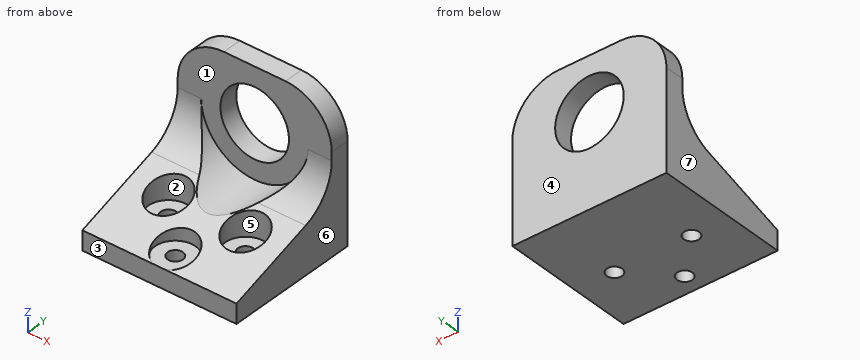
from build123d import *

# Parameters (mm, degrees)
SKETCH1_W           = 50.8
SKETCH1_H           = 44.45
BOSS_EXTRUDE1_DEPTH = 6.35
BOSS_EXTRUDE2_DEPTH = 50.8
SKETCH3_R           = 11.303
CUT_EXTRUDE1_DEPTH  = 50.8
SKETCH4_R           = 2.54
CUT_EXTRUDE2_DEPTH  = 50.8
SKETCH5_R           = 6.6675
CUT_EXTRUDE3_DEPTH  = 41.656
SKETCH6_R           = 17.653
CUT_EXTRUDE4_DEPTH  = 50.8
FILLET1_R           = 15.24


with BuildPart() as part:
    # Sketch1 → Boss-Extrude1 (new body)
    with BuildSketch(Plane.XY):
        with Locations((25.4, 22.225)):
            Rectangle(SKETCH1_W, SKETCH1_H)
    extrude(amount=BOSS_EXTRUDE1_DEPTH)

    # Sketch2 → Boss-Extrude2 (add)
    with BuildSketch(Plane(origin=(50.8, 0, 0), x_dir=(0, 0, -1), z_dir=(1, 0, 0))):
        Polygon((-6.35, 0), (-6.35, 44.45), (-48.006, 44.45), (-48.006, 38.1), (-19.05, 38.1), align=None)
    extrude(amount=-BOSS_EXTRUDE2_DEPTH)

    # Sketch3 → Cut-Extrude1 (cut)
    with BuildSketch(Plane(origin=(0, 44.45, 0), x_dir=(1, 0, 0), z_dir=(0, 1, 0))):
        with Locations(Location((25.4, -30.353, 0), (0, 0, 270))):
            Circle(SKETCH3_R)
    extrude(amount=-CUT_EXTRUDE1_DEPTH, mode=Mode.SUBTRACT)

    # Sketch4 → Cut-Extrude2 (cut)
    with BuildSketch(Plane(origin=(0, 0, 0), x_dir=(-1, 0, 0), z_dir=(0, 0, -1))):
        with Locations((-25.4, 6.35)):
            Circle(SKETCH4_R)
        with Locations((-38.1, 19.05)):
            Circle(SKETCH4_R)
        with Locations((-12.7, 19.05)):
            Circle(SKETCH4_R)
    extrude(amount=-CUT_EXTRUDE2_DEPTH, mode=Mode.SUBTRACT)

    # Sketch5 → Cut-Extrude3 (cut)
    with BuildSketch(Plane.XY.offset(48.006)):
        with Locations((12.7, 19.05)):
            Circle(SKETCH5_R)
        with Locations((38.1, 19.05)):
            Circle(SKETCH5_R)
        with Locations((25.4, 6.35)):
            Circle(SKETCH5_R)
    extrude(amount=-CUT_EXTRUDE3_DEPTH, mode=Mode.SUBTRACT)

    # Sketch6 → Cut-Extrude4 (cut)
    with BuildSketch(Plane.XZ.offset(-38.1)):
        with Locations((25.4, 30.353)):
            Circle(SKETCH6_R)
    extrude(amount=CUT_EXTRUDE4_DEPTH, mode=Mode.SUBTRACT)

    # Fillet1
    fillet1_edges = [part.edges().sort_by_distance(p)[0] for p in [
        (5.92005531, 38.1, 19.05),
        (44.87994469, 38.1, 19.05),
        (50.8, 41.275, 48.006),
        (0, 41.275, 48.006),
    ]]
    fillet(fillet1_edges, radius=FILLET1_R)


solid = part.part
Geometry check sheet. Reference: the model listing, model coordinates, mm. Face numbers are marked on the shaded views. A direction names the side the tool comes from. Give positions to 0.01 mm unless a question says otherwise; leave off trailing zeros. Loops run counter-clockwise (first coordinate to the right, second up) from the corner with the lowest first, then second, coordinate; pieces in that order, holes last. Notation, with made-up numbers: (-22.75, 41.5) -> (28.25, 41.5) arc R23 cw to (28.25, 72.5) -> close; hole circle Ø1 at (74.5, 14.25). An arc over 180 degrees is marked (long way). Answer in a Markdown table with one row per item. Add a question column.
1) Set-up check for the marked faces 1, 2 and 3: record each of +Z, -Z, +X, -X, +Y, -Y from which the full face is reachable in a straight line by a thin tool's end or side.
2) Material ranges on probe 1 along X at (y, z) = (19.05, 11.75); probe 2 along X at (y, z) = (19, 4); probe 3 along X at (y, z) = (6, 7), recorded low to high. Write a range as from..to.
3) Cross-section at C-C on z = 23. Record the boundary of the cut face in (x, y), and give its area (3 significant figures).
4) Gauge pin test, flat ends, axial feed: P1, Ø12, axis at y = 9, z = 18.5, coming from the +X side; P2, Ø3, axis at x = 39, y = 12, coming from the -Z side; P3, Ø4, axis at x = 17.5, y = 22, coming from the +Z side; P4, Ø1, axis at x = 45.5, y = 28, coming from the +Z side. Record the tip position at first contact, or that the pin passes through.
5) Cross-section at A-A on x = 25.4. Record the boundary of the cut face in (y, z), and give its area (3 significant figures).
6) Cross-section at B-B on y = 6.35. Record the boundary of the cut face in (x, z), and give its area (3 significant figures).
7) Draft check along X on the marked faces 4, 5, 6 and 7. Enter one of: pulls with the +X half, pulls with the -X half, needs draft (parallel to the pull), parting line crosses it, or undercut.
8) Cross-section at D-D on x = 38.1. Record the boundary of the cut face in (y, z).
Outcome:
| question | item | result |
|---|---|---|
| 1 | face 1 | +Z, -Y |
| 1 | face 2 | +Z |
| 1 | face 3 | +Z, -Z, +X, -X, -Y |
| 2 | probe 1 | x = 0..6.03, 19.37..31.43, 44.77..50.8 |
| 2 | probe 2 | x = 0..10.16, 15.24..35.56, 40.64..50.8 |
| 2 | probe 3 | x = 0..18.74, 32.06..50.8 |
| 3 | outline | (0, 36.38) -> (9.35, 36.38) -> (9.35, 38.1) -> (16.82, 38.1) -> (16.82, 44.45) -> (0, 44.45) -> close; (33.98, 38.1) -> (41.45, 38.1) -> (41.45, 36.38) -> (50.8, 36.38) -> (50.8, 44.45) -> (33.98, 44.45) -> close |
| 3 | area | 246 mm^2 |
| 4 | P1 | passes through |
| 4 | P2 | stops at z = 0 |
| 4 | P3 | stops at z = 14.35 |
| 4 | P4 | stops at z = 15.88 |
| 5 | outline | (0, 0) -> (3.81, 0) -> (3.81, 6.35) -> (0, 6.35) -> close; (8.89, 0) -> (44.45, 0) -> (44.45, 19.05) -> (38.1, 19.05) -> (38.1, 12.7) -> (19.05, 12.7) -> (13.02, 10.69) -> (13.02, 6.35) -> (8.89, 6.35) -> close; (38.1, 41.66) -> (44.45, 41.66) -> (44.45, 48.01) -> (38.1, 48.01) -> close |
| 5 | area | 524 mm^2 |
| 6 | outline | (0, 0) -> (22.86, 0) -> (22.86, 6.35) -> (18.73, 6.35) -> (18.73, 8.47) -> (0, 8.47) -> close; (27.94, 0) -> (50.8, 0) -> (50.8, 8.47) -> (32.07, 8.47) -> (32.07, 6.35) -> (27.94, 6.35) -> close |
| 6 | area | 370 mm^2 |
| 7 | face 4 | needs draft |
| 7 | face 5 | undercut |
| 7 | face 6 | pulls with the +X half |
| 7 | face 7 | pulls with the -X half |
| 8 | outline | (0, 0) -> (16.51, 0) -> (16.51, 6.35) -> (12.38, 6.35) -> (12.38, 10.48) -> (0, 6.35) -> close; (21.59, 0) -> (44.45, 0) -> (44.45, 47.79) -> (38.1, 47.79) -> (38.1, 18.09) -> (32.33, 18.09) arc R15.24 cw to (27.68, 15.58) -> (25.72, 14.92) -> (25.72, 6.35) -> (21.59, 6.35) -> close |
